Autodesk Inventor part; units mm, degrees
ref_plane "Work Plane1" through (0, 40, -50.485) normal (0, 0, -1) x (-1, 0, 0)
ref_plane "YZ Plane" through (0, 0, 0) normal (1, 0, 0) x (0, 1, 0)
ref_plane "XZ Plane" through (0, 0, 0) normal (0, 1, 0) x (-1, 0, 0)
sketch "Sketch1" plane through (0, 0, 0) normal (0, 1, 0) x (-1, 0, 0)
  circle A0 centre (0, 0) radius 67.5
  dimension "d0" = 135
extrude "body" add sketch "Sketch1" along normal blind 40
sketch "Sketch2" plane through (0, 40, 0) normal (0, 1, 0) x (1, 0, 0)
  circle A0 centre (0, 0) radius 67.5
  circle A1 centre (0, 0) radius 45.085
  dimension "d4" = 90.17
extrude "hole" cut sketch "Sketch2" against normal blind 101.6 contours A1
sketch "Sketch3" plane through (0, 40, 0) normal (0, 1, 0) x (1, 0, 0)
  circle A0 centre (0, 0) radius 45.085
  circle A1 centre (0, 0) radius 67.5
  circle A2 centre (0, 0) radius 50.485
  dimension "d9" = 5.4
extrude "flange" cut sketch "Sketch3" against normal blind 34 contours A1
sketch "Sketch4" plane through (0, 40, 0) normal (0, 1, 0) x (1, 0, 0)
  circle A0 centre (0, 0) radius 50.485
  circle A1 centre (0, 0) radius 45.085
  point P0 (0, 50.485)
ref_plane "Work Plane1" through (0, 40, -50.485) normal (0, 0, -1) x (-1, 0, 0)
sketch "Sketch5" plane through (0, 40, -50.485) normal (0, 0, -1) x (-1, 0, 0)
  circle A0 centre (0, -13) radius 2.54
  line L0 (50.485, 0) -> (-50.485, 0)
  point P0 (0, -40)
  dimension "d12" = 13
  dimension "d13" = 5.08
hole "sideHoleSE" at (0, 27, -50.485) direction (0, 0, 1) diameter 4.1402 depth 25.4 tip angle 118
pattern_circular "sideHoleSW" count 2 over 120 about axis through (0, 40, 0) along (0, -1, 0) of "sideHoleSE"
pattern_circular "sideHoleN" count 2 over 130 about axis through (0, 40, 0) along (0, 1, 0) of "sideHoleSE"
sketch "Sketch8" plane through (0, 6, 0) normal (0, 1, 0) x (1, 0, 0)
  circle A0 centre (0, 0) radius 50.485
  circle A1 centre (0, 0) radius 67.5
  circle A2 centre (0, 57) radius 3.1903
  line L0 (0, 0) -> (49.3634, -28.5) construction
  line L1 (0, 0) -> (57, 0) construction
  circle A3 centre (49.3634, -28.5) radius 3.101
  line L2 (0, 0) -> (-51.9615, -30) construction
  line L3 (0, 0) -> (60, 0) construction
  circle A4 centre (-51.9615, -30) radius 3.5807
  dimension "d65" = 57
  dimension "d66" = 57
  dimension "d67" = 30
  dimension "d68" = 60
  dimension "d69" = 150
hole "Hole5" at (0, 6, -57) at (49.3634, 6, 28.5) at (-51.9615, 6, 30) direction (0, -1, 0) diameter 6.6 end through all
properties part number "2f1col" material "Aluminum 6061"
Source: CAD feature listing. Evaluate the final solid. Frame: model axes, mm. A direction names the side the tool comes from. Give positions to 0.01 mm unless a question says otherwise; leave off trailing zeros. Write each loop counter-clockwise with the first axis right and the second up, starting at its lowest first coordinate (ties: lowest second). Pieces come first, ordered by that corner, then holes. Notation, with made-up numbers: (-15, 33.25) -> (1, 33.25) arc R22 ccw to (1, 45.25) -> close; hole circle Ø3 at (24.25, -29.75). An arc over 180 degrees is marked (long way). Return JSON: item names as keys, results as strings. Group by question number.
1. Section C-C, the plane y = 36.5. Output: boundary loops of the cut face in (x, z) (3 decimals), then the cut area to 3 significant figures.
2. Material intervals for line 1 (Z direction, x = 0, y = 1.6) (3 decimals); line 2 (Z direction, x = 0, y = 17.5) (3 decimals); line 3 (X direction, y = 3, z = 28.5), sorted ascending. Write a range as from..to.
3. Mould query, pull axis Y, two halves, no side actions, for faces 1 (the face through (52.291, 2.958, 30.023)), 2 (the face through (-44, 0, -14)), 3 (the face through (-0.09, 24.93, -47.72)). Classes: +Y half, -Y half, draft (parallel to the pull), parting line (faces both ways), or undercut.
4. Pin query (flat end, axial travel): pin 1 Ø1 at (x, y) = (18.5, 22) entering from -Z; pin 2 Ø4 at (y, z) = (24, 23.5) entering from -X; pin 3 Ø5 at (x, y) = (-21.5, 12.5) entering from +Z; pin 4 Ø8 at (x, z) = (-45, 34.5) entering from -Y. Return the tip coordinate at first contact, or that it passes through.
5. Access query for faces 4 (the face through (-10.944, 23.238, 49.284)), 5 (the face through (18.9, 40, 41.4)). Directions: +Z, -Z, +X, -X, +Y, -Y. A direction counts if a zero-diameter tool reaches every point of the face in a straight line with its end or side. Return the directions, or none.
6. Section A-A, the plane x = 0. Output: boundary loops of the cut face in (y, z) (3 decimals), then the cut area to 3 significant figures.
7. Section D-D, the plane x = 41. Count the separate pieces of the cut face and the enclosed holes in it, then the cut area to 3 significant figures.
8. Section B-B, the plane z = 0. Output: boundary loops of the cut face in (x, y) (3 decimals), then the cut area to 3 significant figures.
Determined:
{
 "1": {"outline": "circle Ø100.97 at (0, 0); hole circle Ø90.17 at (0, 0)", "area": "1,620 mm2"},
 "2": {"line 1": "z = -67.5..-60.3, -53.7..-45.085, 45.085..67.5", "line 2": "z = -50.485..-45.085, 45.085..50.485", "line 3": "x = -61.19..-54.9, -49.02..-34.93, 34.93..46.06, 52.66..61.19"},
 "3": {"face 1": "draft", "face 2": "-Y half", "face 3": "undercut"},
 "4": {"pin 1": "stops at z = -47.17", "pin 2": "stops at x = -45.68", "pin 3": "stops at z = 46.77", "pin 4": "stops at y = 0"},
 "5": {"face 4": "+Y", "face 5": "+Z, -Z, +X, -X, +Y"},
 "6": {"outline": "(0, -67.5) -> (6, -67.5) -> (6, -60.3) -> (0, -60.3) -> close; (0, -53.7) -> (6, -53.7) -> (6, -50.485) -> (24.93, -50.485) -> (24.93, -45.085) -> (0, -45.085) -> close; (0, 45.085) -> (40, 45.085) -> (40, 50.485) -> (6, 50.485) -> (6, 67.5) -> (0, 67.5) -> close; (29.07, -50.485) -> (40, -50.485) -> (40, -45.085) -> (29.07, -45.085) -> close", "area": "574 mm2"},
 "7": {"separate pieces": "2", "enclosed holes": "1", "area": "1,130 mm2"},
 "8": {"outline": "(-67.5, 0) -> (-45.085, 0) -> (-45.085, 40) -> (-50.485, 40) -> (-50.485, 6) -> (-67.5, 6) -> close; (45.085, 0) -> (67.5, 0) -> (67.5, 6) -> (50.485, 6) -> (50.485, 40) -> (45.085, 40) -> close", "area": "636 mm2"}
}
